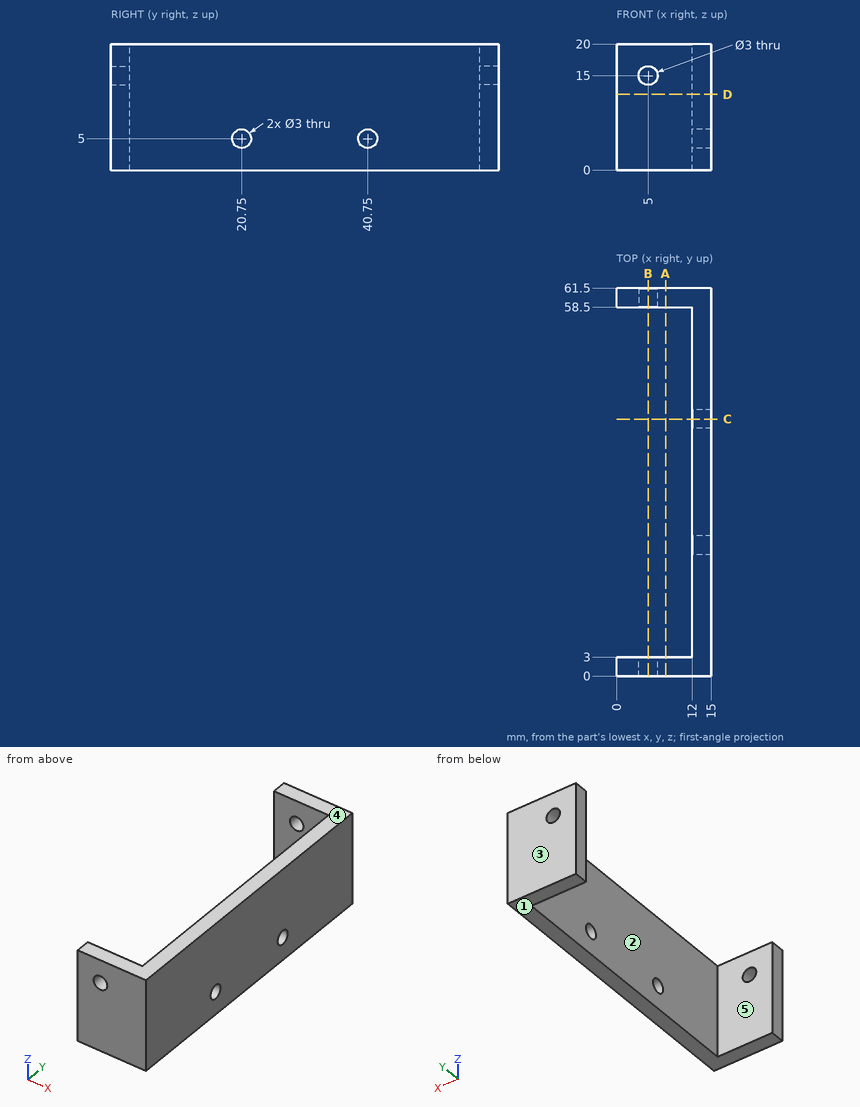
Drawing for the job (mm, zero at the part's lowest x, y, z). A direction names the side the tool comes from. Give positions to 0.01 mm unless a question says otherwise; leave off trailing zeros. Loops run counter-clockwise (first coordinate to the right, second up) from the corner with the lowest first, then second, coordinate; pieces in that order, holes last. Notation, with made-up numbers: (44, 16) - (100, 16) arc R32 ccw to (100, 44) - close; hole circle Ø2 at (42, 66). An arc over 180 degrees is marked (long way). Write item = value, one per line. Start each with the question number.
1) Pull direction Y, two halves, no side cores. Call the marked faces 1, 2 and 3: +Y half, -Y half, draft (parallel to the pull), parting line (faces both ways), or undercut.
2) Band-saw the part on A-A on x = 7.75. Give the cut face in (y, z), plus the area to 3 significant figures.
3) Probe probe 1 along Y at (x, z) = (12.95, 5); probe 2 along X at (y, z) = (1.7, 15); probe 3 along Y at (x, z) = (3.75, 2.75). List the from-to ranges inside material, lowest first. Write a range as from..to.
4) Band-saw the part on B-B on x = 5. Give the cut face in (y, z), plus the area to 3 significant figures.
5) Band-saw the part on C-C on y = 40.75. Give the cut face in (x, z), plus the area to 3 significant figures.
6) Band-saw the part on D-D on z = 12. Give the cut face in (x, y), plus the area to 4 significant figures.
7) Drop flat-ended pins along their axis: pin 1 Ø2.5 at (y, z) = (40.75, 5) entering from -X; pin 2 Ø3 at (y, z) = (12, 11.5) entering from -X. Give the stop position or say it passes through.
8) Tool access for the marked faces 4 and 5: list every direction of +Z, -Z, +X, -X, +Y, -Y with a clear straight run to the whole face (end or side of a thin tool).
Final values:
q1.face_1 = draft
q1.face_2 = undercut
q1.face_3 = +Y half
q2.outline = (0, 0) - (3, 0) - (3, 20) - (0, 20) - close; (58.5, 0) - (61.5, 0) - (61.5, 20) - (58.5, 20) - close
q2.area = 120 mm²
q3.probe_1 = 0..19.25, 22.25..39.25, 42.25..61.5
q3.probe_2 = 0..3.5, 6.5..15
q3.probe_3 = 0..3, 58.5..61.5
q4.outline = (0, 0) - (3, 0) - (3, 13.5) - (0, 13.5) - close; (0, 16.5) - (3, 16.5) - (3, 20) - (0, 20) - close; (58.5, 0) - (61.5, 0) - (61.5, 13.5) - (58.5, 13.5) - close; (58.5, 16.5) - (61.5, 16.5) - (61.5, 20) - (58.5, 20) - close
q4.area = 102 mm²
q5.outline = (12, 0) - (15, 0) - (15, 3.5) - (12, 3.5) - close; (12, 6.5) - (15, 6.5) - (15, 20) - (12, 20) - close
q5.area = 51.0 mm²
q6.outline = (0, 0) - (15, 0) - (15, 61.5) - (0, 61.5) - (0, 58.5) - (12, 58.5) - (12, 3) - (0, 3) - close
q6.area = 256.5 mm²
q7.pin_1 = through
q7.pin_2 = 12
q8.face_4 = +Z, +X, -X, +Y, -Y
q8.face_5 = +Z, -Z, -X
